```python
from build123d import *

# Parameters (mm, degrees)
F0_R          = 44.45
F1_DEPTH      = 95.25
F2_T          = -5.08
F3_R          = 3.175
F4_DEPTH      = 44.451
F4_DEPTH_BACK = 44.451


with BuildPart() as f1:
    # F0 (on Top) → F1 (new body)
    with BuildSketch(Plane.XY):
        Circle(F0_R)
    extrude(amount=F1_DEPTH)

    # F2
    f2_openings = [f1.faces().sort_by_distance(p)[0] for p in [
        (0, 0, 95.25),
    ]]
    offset(amount=F2_T, openings=f2_openings)

    # F3 (on Front) → F4 (cut, two sides)
    with BuildSketch(Plane.XZ) as f4_sk:
        with Locations((0, 86.995)):
            Circle(F3_R)
    extrude(amount=-F4_DEPTH, mode=Mode.SUBTRACT)
    extrude(f4_sk.sketch, amount=F4_DEPTH_BACK, mode=Mode.SUBTRACT)


solid = f1.part
```
Could you check a few things on this model? Use its own coordinates, in mm. A direction names the side the tool comes from. Coordinates: 2 decimals unless noted, no trailing zeros. Write each loop counter-clockwise with the first axis right and the second up, starting at its lowest first coordinate (ties: lowest second). Pieces come first, ordered by that corner, then holes. Notation, with made-up numbers: (43, -0.75) -> (63, -0.75) arc R27 cw to (63, 33.25) -> close; hole circle Ø11 at (56.25, 63.25). An arc over 180 degrees is marked (long way). Write item = value, one per line. Start each with the question number.
(1) I want a section at C-C (y = 27.5). Please give me the cut outline in (x, z).
(2) Will these pins go through, and if not, where does the flat tip stop? pin 1 (1 mm diameter, centred on x = -6.5, z = 84.5, fed in from +Y); pin 2 (10 mm diameter, centred on x = -31.5, z = 65, fed in from -Y); pin 3 (8 mm diameter, centred on y = -24, z = 15, fed in from +X).
(3) I want a section at D-D (x = -34). Please give me the cut outline in (y, z).
(4) I want a section at A-A (x = 0). Please give me the cut outline in (y, z).
(5) Which directions (+Z, -Z, +X, -X, +Y, -Y) give clear straight access to the entire face, cutting with the end or side of a thin tool? Please do faces 4 (the face through (-39.33, 1.73, 49.53)), 5 (the face through (-27, -29, 95.25)).
(6) I need wall thicknesses on line 1 (Z direction, x = 0, y = -42); line 2 (Y direction, x = 0, z = 76); line 3 (Y direction, x = -22.5, z = 54). Which ranges of each line are inside material? Lowest first, please. Write a range as [from, to].
(7) We'd pull the mould along X, two halves only. Please class faces 1 (the face through (-2.34, 41.81, 89.14)), 2 (the face through (42.397, 13.352, 46.958)), 3 (the face through (-1, 1, 0)): released by +X, released by -X, zero draft, split by the parting line, or undercut.
(8) I want a section at B-B (z = 73). Please give me the cut outline in (x, y), plus the area to 3 significant figures.
Result set:
q1.outline = (-34.92, 0) -> (34.92, 0) -> (34.92, 95.25) -> (28.17, 95.25) -> (28.17, 5.08) -> (-28.17, 5.08) -> (-28.17, 95.25) -> (-34.92, 95.25) -> close
q2.pin_1 = 44.04
q2.pin_2 = -35.69
q2.pin_3 = 39.7
q3.outline = (-28.63, 0) -> (28.63, 0) -> (28.63, 95.25) -> (19.85, 95.25) -> (19.85, 5.08) -> (-19.85, 5.08) -> (-19.85, 95.25) -> (-28.63, 95.25) -> close
q4.outline = (-44.45, 0) -> (44.45, 0) -> (44.45, 83.82) -> (39.37, 83.82) -> (39.37, 5.08) -> (-39.37, 5.08) -> (-39.37, 83.82) -> (-44.45, 83.82) -> close; (-44.45, 90.17) -> (-39.37, 90.17) -> (-39.37, 95.25) -> (-44.45, 95.25) -> close; (39.37, 90.17) -> (44.45, 90.17) -> (44.45, 95.25) -> (39.37, 95.25) -> close
q5.face_4 = +Z
q5.face_5 = +Z, +X, -X, +Y, -Y
q6.line_1 = [0, 83.82], [90.17, 95.25]
q6.line_2 = [-44.45, -39.37], [39.37, 44.45]
q6.line_3 = [-38.33, -32.31], [32.31, 38.33]
q7.face_1 = undercut
q7.face_2 = split by the parting line
q7.face_3 = zero draft
q8.outline = circle Ø88.9 at (0, 0); hole circle Ø78.74 at (0, 0)
q8.area = 1,340 mm2
